```python
from build123d import *

# Parameters (mm, degrees)
SZKIC1_W                        = 40
SZKIC1_H                        = 40
DODANIE_WYCI_GNI_CIE1_DEPTH     = 80
WYTNIJ_WYCI_GNI_CIE2_DEPTH      = 85.852813742
WYTNIJ_WYCI_GNI_CIE2_DEPTH_BACK = 80
SZKIC3_R                        = 4
WYTNIJ_WYCI_GNI_CIE3_DEPTH      = 91.382520434


with BuildPart() as part:
    # Szkic1 → Dodanie-wyciągnięcie1 (new body)
    with BuildSketch(Plane(origin=(0, 0, 0), x_dir=(1, 0, 0), z_dir=(0, 1, 0))):
        Rectangle(SZKIC1_W, SZKIC1_H)
    extrude(amount=DODANIE_WYCI_GNI_CIE1_DEPTH)

    # Szkic2 → Wytnij-wyciągnięcie2 (cut, two sides: drawn at the far end of the back side and taken through both)
    with BuildSketch(Plane(origin=(0, 80, 0), x_dir=(1, 0, 0), z_dir=(0, 1, 0)).offset(-WYTNIJ_WYCI_GNI_CIE2_DEPTH_BACK)):
        Polygon((-17, 0), (-17, -20), (20, -20), (20, 17), (0, 17), align=None)
    extrude(amount=WYTNIJ_WYCI_GNI_CIE2_DEPTH + WYTNIJ_WYCI_GNI_CIE2_DEPTH_BACK, mode=Mode.SUBTRACT)

    # Szkic3 → Wytnij-wyciągnięcie3 (cut, through all)
    with BuildSketch(Plane.XY.offset(-17)):
        with Locations((10, 60)):
            Circle(SZKIC3_R)
        with Locations(Location((10, 20, 0), (0, 0, 180))):
            Circle(SZKIC3_R)
    wytnij_wyci_gni_cie3 = extrude(amount=-WYTNIJ_WYCI_GNI_CIE3_DEPTH, mode=Mode.SUBTRACT)

    # Lustro1: Wytnij-wyciągnięcie3 across plane
    add(wytnij_wyci_gni_cie3.mirror(Plane(origin=(0, 0, 0), x_dir=(0.7071067811865476, 0, 0.7071067811865475), z_dir=(-0.7071067811865475, 0, 0.7071067811865476))), mode=Mode.SUBTRACT)


solid = part.part
```
Model file for the job. Use its own axes, mm. A direction names the side the tool comes from. Give positions to 0.01 mm unless a question says otherwise; leave off trailing zeros. Order: outer loops, then holes, each group sorted by start corner. A loop starts at its lowest first (then second) coordinate and runs counter-clockwise, first axis right, second up.
1) 3-axis set-ups, long thin cutter, end or side, ignore diameter. For faces 1 (the flat face through (-19, 39, 20)), 2 (the flat face through (10, 39, -17)): which of +Z, -Z, +X, -X, +Y, -Y reach the whole face in a straight line?
2) Wall check: probe 1 along Y at (x, z) = (-18.85, 10); probe 2 along X at (y, z) = (20, -19). Give the ranges that are in metal, low to high.
3) Saw through at D-D, the plane z = 1. Write the cut outline in (x, y), then the cut area to 3 significant figures.
4) Mould opens along X. For faces 3 (the cylindrical face through (-18.479, 56.095, 9.133)), 4 (the cylindrical face through (12.95, 17.3, -18.48)), 5 (the flat face through (-8, 39, -9)) say: +X half, -X half, draft (parallel to the pull), parting line (faces both ways), or undercut.
5) Saw through at A-A, the plane z = 10. Write the cut outline in (x, y), then the cut area to 3 significant figures.
6) Pin check, flat tips, straight feed: pin 1 (13 mm diameter, centred on y = 60, z = 10, fed in from +X); pin 2 (10 mm diameter, centred on x = 5.5, y = 27.5, fed in from +Z); pin 3 (10 mm diameter, centred on x = -0.5, z = -2.5, fed in from -Y). Stop position of each tip, or through.
7) Saw through at B-B, the plane y = 60. Write the cut outline in (x, z), then the cut area to 4 significant figures.
8) Saw through at C-C, the plane x = 10.5. Write the cut outline in (y, z).
Computed:
1. face 1: +Z, +X, -X, +Y, -Y
1. face 2: +Z, +X, +Y, -Y
2. probe 1: y = 0 to 16, 24 to 56, 64 to 80
2. probe 2: x = -20 to 6, 14 to 20
3. outline: (-20, 0) - (-17, 0) - (-17, 80) - (-20, 80) - close
3. area: 240 mm2
4. face 3: draft
4. face 4: undercut
4. face 5: +X half
5. outline: (-20, 0) - (-17, 0) - (-17, 16) - (-20, 16) - close; (-20, 24) - (-17, 24) - (-17, 56) - (-20, 56) - close; (-20, 64) - (-17, 64) - (-17, 80) - (-20, 80) - close
5. area: 192 mm2
6. pin 1: stops at x = -17
6. pin 2: stops at z = -17
6. pin 3: passes through
7. outline: (-20, -20) - (6, -20) - (6, -17) - (0, -17) - (-17, 0) - (-17, 6) - (-20, 6) - close; (-20, 14) - (-17, 14) - (-17, 20) - (-20, 20) - close; (14, -20) - (20, -20) - (20, -17) - (14, -17) - close
7. area: 327.5 mm2
8. outline: (0, -20) - (16.03, -20) - (16.03, -17) - (0, -17) - close; (23.97, -20) - (56.03, -20) - (56.03, -17) - (23.97, -17) - close; (63.97, -20) - (80, -20) - (80, -17) - (63.97, -17) - close
